```python
from build123d import *

# Parameters (mm, degrees)
BODY_SKETCH_R      = 2.45
BASE_FLANGE1_DEPTH = 0.5


# Sheet-metal steps are written as plain solids
with BuildPart() as part:
    # Body Sketch → Base-Flange1 (new body)
    with BuildSketch(Plane.XY):
        with BuildLine():
            Line((2.961840644, 2.3), (10, 2.3))
            Line((10, 2.3), (10, -2.3))
            Line((10, -2.3), (2.961840644, -2.3))
            ThreePointArc((2.961840644, -2.3), (-3.75, 0), (2.961840644, 2.3))
        make_face()
        Circle(BODY_SKETCH_R, mode=Mode.SUBTRACT)
    extrude(amount=-BASE_FLANGE1_DEPTH)


solid = part.part
```
For this review, take the finished solid that the model builds, in its own axes (mm). Give positions to 0.01 mm unless a question says otherwise; leave off trailing zeros. Write each loop counter-clockwise with the first axis right and the second up, starting at its lowest first coordinate (ties: lowest second). Pieces come first, ordered by that corner, then holes. Notation, with made-up numbers: M 31,-25 L 50,-25 A12 ccw 50,-7 Z; hole C 84.25,-10 d1. An arc over 180 degrees is marked long. One line per item, written item: value.
1) The part is to be moulded in two halves that separate along Y. For faces 1 (the flat face through (3, 0, -0.5)), 2 (the cylindrical face through (-0.5, -2.4, -0.2)), 3 (the cylindrical face through (-3.748, -0.13, -0.246)), say which applies: +Y half, -Y half, draft (parallel to the pull), parting line (faces both ways), or undercut.
Results are:
face 1: draft
face 2: undercut
face 3: parting line
2) For P1, Ø4, axis at x = 5.5, y = -1.5, coming from the +Z side, flat-tipped, find the tip position at first contact; note if it passes through.
Results are:
P1: stops at z = 0
3) For line 1 (Y direction, x = 0, z = -0.3); line 2 (Y direction, x = 7.75, z = -0.25); line 3 (X direction, y = -0.5, z = -0.1), list the stretches that pass through material, from the lowest coordinate up. Write a range as from..to.
Results are:
line 1: y = -3.75..-2.45, 2.45..3.75
line 2: y = -2.3..2.3
line 3: x = -3.72..-2.4, 2.4..10
4) Take a section at A-A, the plane x = 0. Write out the cut boundary in (y, z), then the cut area to 3 significant figures.
Results are:
outline: M -3.75,-0.5 L -2.45,-0.5 L -2.45,0 L -3.75,0 Z; M 2.45,-0.5 L 3.75,-0.5 L 3.75,0 L 2.45,0 Z
area: 1.30 mm²
5) Take a section at C-C, the plane z = -0.25. Write out the cut boundary in (x, y), then the cut area to 3 significant figures.
Results are:
outline: M 2.96,-2.3 L 10,-2.3 L 10,2.3 L 2.96,2.3 A3.75 ccw long Z; hole C 0,0 d4.9
area: 55.2 mm²
6) Take a section at B-B, the plane y = 1.5. Write out the cut boundary in (x, z), then the cut area to 3 significant figures.
Results are:
outline: M -3.44,-0.5 L -1.94,-0.5 L -1.94,0 L -3.44,0 Z; M 1.94,-0.5 L 10,-0.5 L 10,0 L 1.94,0 Z
area: 4.78 mm²
